Geometry check sheet. Reference: the model listing, model coordinates, mm. A direction names the side the tool comes from. Round coordinates to 2 decimals unless told otherwise and drop trailing zeros. Write each loop counter-clockwise with the first axis right and the second up, starting at its lowest first coordinate (ties: lowest second). Pieces come first, ordered by that corner, then holes.
Item 1: Cross-section at B-B (x = 15). Enter the section's corners in (y, z), then the cut area to 3 significant figures.
Item 2: Cross-section at D-D (z = 9.75). Enter the section's corners in (x, y).
Item 3: Cross-section at C-C (y = 42). Enter the section's corners in (x, z), then the cut area to 3 significant figures.
Item 4: Scan lines: probe 1 along Y at (x, z) = (3.5, 0); probe 2 along X at (y, z) = (47, -2.75). Record each from-to range of solid material in increasing order.
Item 5: Cross-section at A-A (z = 0). Enter the section's corners in (x, y), then the cut area to 3 significant figures.
Item 6: Draft check along Y on faces 3 (the face through (3.944, 45.074, -0.404)), 4 (the face through (27, 0, 0)), 5 (the face through (8, 45.4, 0.2)), 6 (the face through (20, 21, 0)). Enter one of: pulls with the +Y half, pulls with the -Y half, needs draft (parallel to the pull), parting line crosses it, or undercut.
Item 7: Access from +Z, -Z, +X, -X, +Y, -Y to the whole of each face (thin tool, end or side, straight path). Record for faces 1 (the face through (17, 13, -11)), 2 (the face through (45, 8, 3)).
Item 8: Depth check by flat-ended pin: P1, Ø2, axis at x = 29.5, z = -0.5, coming from the +Y side; P2, Ø6, axis at x = 44, y = 12, coming from the -Z side; P3, Ø6, axis at x = 44.5, z = 4, coming from the +Y side; P4, Ø1.5, axis at y = 40.5, z = -6, coming from the +X side. Enter the tip coordinate at first touch or a pass-through.
from build123d import *

# Parameters (mm, degrees)
SKETCH_1_R              = 2.3
EXTRUDE_1_DEPTH         = 11
HOLE_WIZARD_6_2_6_2_1_D = 6.2
HOLE_WIZARD_6_2_6_2_2_D = 6.2


with BuildPart() as part:
    # 草图1 → 凸台-拉伸1 (new, symmetric)
    with BuildSketch(Plane.XY):
        Polygon((0, 0), (0, 53), (8, 53), (8, 33), (33, 8), (53, 8), (53, 0), align=None)
        with Locations((15, 15)):
            Circle(SKETCH_1_R, mode=Mode.SUBTRACT)
    extrude(amount=EXTRUDE_1_DEPTH, both=True)

    # Ø6.2 (6.2) 直径孔1 (through all)
    with Locations(Plane(origin=(0, 8, 0), x_dir=(1, 0, 0), z_dir=(0, 1, 0))):
        with Locations((42, 0)):
            Hole(HOLE_WIZARD_6_2_6_2_1_D / 2)

    # Ø6.2 (6.2) 直径孔2 (through all)
    with Locations(Plane(origin=(8, 0, 0), x_dir=(0, 0, -1), z_dir=(1, 0, 0))):
        with Locations((0, 42)):
            Hole(HOLE_WIZARD_6_2_6_2_2_D / 2)


solid = part.part
Resolved:
1. outline: (0, -11) - (12.7, -11) - (12.7, 11) - (0, 11) - close; (17.3, -11) - (26, -11) - (26, 11) - (17.3, 11) - close
1. area: 471 mm2
2. outline: (0, 0) - (53, 0) - (53, 8) - (33, 8) - (8, 33) - (8, 53) - (0, 53) - close; hole circle Ø4.6 at (15, 15)
3. outline: (0, -11) - (8, -11) - (8, -3.1) - (0, -3.1) - close; (0, 3.1) - (8, 3.1) - (8, 11) - (0, 11) - close
3. area: 126 mm2
4. probe 1: y = 0 to 38.9, 45.1 to 53
4. probe 2: x = 0 to 8
5. outline: (0, 0) - (38.9, 0) - (38.9, 8) - (33, 8) - (8, 33) - (8, 38.9) - (0, 38.9) - close; (0, 45.1) - (8, 45.1) - (8, 53) - (0, 53) - close; (45.1, 0) - (53, 0) - (53, 8) - (45.1, 8) - close; hole circle Ø4.6 at (15, 15)
5. area: 981 mm2
6. face 3: undercut
6. face 4: pulls with the -Y half
6. face 5: needs draft
6. face 6: pulls with the +Y half
7. face 1: -Z, +X, -X, +Y, -Y
7. face 2: +Z, -Z, +X, +Y
8. P1: stops at y = 12.5
8. P2: passes through
8. P3: stops at y = 8
8. P4: stops at x = 8
